from build123d import *

# Parameters (mm, degrees)
SKETCH2_W          = 16.5
SKETCH2_H          = 15.5
SKETCH2_W_2        = 14.5
SKETCH2_H_2        = 3.4
CUT_EXTRUDE1_DEPTH = 2.3


with BuildPart() as part:
    # Sketch1 → Revolve1 (revolve)
    with BuildSketch(Plane.XY):
        Polygon((0, 7.05), (0, 3), (7.7, 3), (7.7, 7.25), (0.2, 7.25), align=None)
    revolve(axis=Axis((7.7, 0, 0), (-1, 0, 0)))

    # Sketch2 → Cut-Extrude1 (cut)
    with BuildSketch(Plane(origin=(7.7, 0, 0), x_dir=(0, 0, -1), z_dir=(1, 0, 0))):
        Rectangle(SKETCH2_W, SKETCH2_H)
        Rectangle(SKETCH2_W_2, SKETCH2_H_2, mode=Mode.SUBTRACT)
    extrude(amount=-CUT_EXTRUDE1_DEPTH, mode=Mode.SUBTRACT)

    # Sketch3 → Cut-Revolve1 (revolve, cut)
    with BuildSketch(Plane(origin=(2.6, 0, 0), x_dir=(0, 0, -1), z_dir=(1, 0, 0))):
        Polygon((-7.25, 0), (-7.25, 1.5), (-6.9795, 1.2295), (0, 1.2295), (0, 0), align=None)
    revolve(axis=Axis((2.6, 0, 0), (0, 0, 1)), mode=Mode.SUBTRACT)

    # Sketch4 → Cut-Revolve2 (revolve, cut)
    with BuildSketch(Plane(origin=(2.6, 0, 0), x_dir=(0, 0, -1), z_dir=(1, 0, 0))):
        Polygon((0, -7.25), (-1.5, -7.25), (-1.2295, -6.9795), (-1.2295, 0), (0, 0), align=None)
    revolve(axis=Axis((2.6, 0, 0), (0, -1, 0)), mode=Mode.SUBTRACT)


solid = part.part
For this review, take the finished solid that the model builds, in its own axes (mm). A direction names the side the tool comes from. Round coordinates to 2 decimals unless told otherwise and drop trailing zeros. Loops run counter-clockwise (first coordinate to the right, second up) from the corner with the lowest first, then second, coordinate; pieces in that order, holes last. Notation, with made-up numbers: (30.25, 25) - (63.25, 25) arc R12 ccw to (63.25, 36) - close; hole circle Ø1 at (78.5, 16). An arc over 180 degrees is marked (long way). Put each result on its own line as item: value. Start each with the question number.
1. Consider section A-A on z = 0. State the section outline as (x, y) points, plus the area to 3 significant figures.
2. For faces 1 (the flat face through (5.4, 4, 0)), 2 (the cylindrical face through (1.38, -4.83, -0.16)), 3 (the flat face through (7, -1.7, 5)), list the 3-axis set-ups (+Z, -Z, +X, -X, +Y, -Y) from which the entire face can be reached by the end or side of a thin tool; tool diameter is ignored.
3. Mouldability with a two-part tool opening along Z and no side actions: class faces 4 (the cylindrical face through (3.064, 6.697, 2.777)), 5 (the cylindrical face through (3.05, 2.86, -0.9)), 6 (the flat face through (7.7, 0, -5)) as +Z half, -Z half, draft (parallel to the pull), parting line (faces both ways), or undercut.
4. Consider section C-C on y = 0. State the section outline as (x, z) points.
5. For probe 1 along X at (y, z) = (-4.1, 0); probe 2 along X at (y, z) = (-5, 4.5); probe 3 along Y at (x, z) = (1.5, 2.25), list the stretches that pass through material, from the lowest coordinate up. Write a range as [from, to].
6. Consider section D-D on x = 4.5. State the section outline as (y, z) points.
7. Insertion check: P1, Ø4, axis at x = 2.6, y = 0, coming from the +Z side; P2, Ø1.8, axis at x = 7, z = -6, coming from the -Y side; P3, Ø2, axis at x = 2.6, z = 0, coming from the -Y side; P4, Ø2, axis at x = 3.5, z = -3, coming from the +Y side. Each pin has a flat end and moves straight along its axis. Give the tip position at first contact, or say it passes through.
8. Consider section B-B on x = 7.25. State the section outline as (y, z) points, plus the area to 3 significant figures.
Result sheet:
1. outline: (0, -7.05) - (0.2, -7.25) - (1.1, -7.25) - (1.37, -6.98) - (1.37, -3) - (0, -3) - close; (0, 3) - (5.4, 3) - (5.4, 7.25) - (0.2, 7.25) - (0, 7.05) - close; (3.83, -6.98) - (4.1, -7.25) - (5.4, -7.25) - (5.4, -3) - (3.83, -3) - close
1. area: 35.3 mm^2
2. face 1: +Z, -Z, +X, +Y
2. face 2: -Y
2. face 3: +Z, -Z, +X, -Y
3. face 4: parting line
3. face 5: undercut
3. face 6: draft
4. outline: (0, -7.05) - (0.2, -7.25) - (7.7, -7.25) - (7.7, -3) - (0, -3) - close; (0, 3) - (1.37, 3) - (1.37, 6.98) - (1.1, 7.25) - (0.2, 7.25) - (0, 7.05) - close; (3.83, 3) - (7.7, 3) - (7.7, 7.25) - (4.1, 7.25) - (3.83, 6.98) - close
5. probe 1: [0, 1.37], [3.83, 5.4]
5. probe 2: [0, 5.4]
5. probe 3: [-6.89, -1.98], [1.98, 6.89]
6. outline: circle Ø14.5 at (0, 0); hole circle Ø6 at (0, 0)
7. P1: z = 7.25
7. P2: y = -1.7
7. P3: y = 2.83
7. P4: y = 6.97
8. outline: (-1.7, -7.05) arc R7.25 ccw to (1.7, -7.05) - (1.7, -2.47) arc R3 cw to (-1.7, -2.47) - close; (-1.7, 2.47) arc R3 cw to (1.7, 2.47) - (1.7, 7.05) arc R7.25 ccw to (-1.7, 7.05) - close
8. area: 29.6 mm^2
